Job drawing, mm, ordinate dimensions from the low corner. One solid piece. Coordinates: 2 decimals unless noted, no trailing zeros. Loops run counter-clockwise (first coordinate to the right, second up) from the corner with the lowest first, then second, coordinate; pieces in that order, holes last. Notation, with made-up numbers: M 31,-38 L 69,-38 A21 ccw 69,-27 Z; hole C 25,37 d9. An arc over 180 degrees is marked long. Answer as a JSON object with one key per item and string values. Group by question number.
1. Mould opens along X. For the marked faces 1, 2, 3 and 4 say: released by +X, released by -X, zero draft, split by the parting line, or undercut.
2. Saw through at B-B on y = 0.55. Write the cut outline in (x, z).
3. Saw through at C-C on x = 5.25. Write the cut outline in (y, z), then the cut area to 3 significant figures.
4. Drill centre lines: L1, parallel to X at y = 0.2, z = 9.25; L2, parallel to X at y = 2.65, z = 9 (1 decimal); L3, parallel to Z at x = 4.5, y = 1.4 (1 decimal). Where is each one in solid material? Low to high.
5. Saw through at A-A on x = 4.15. Write the cut outline in (y, z), then the cut area to 3 significant figures.
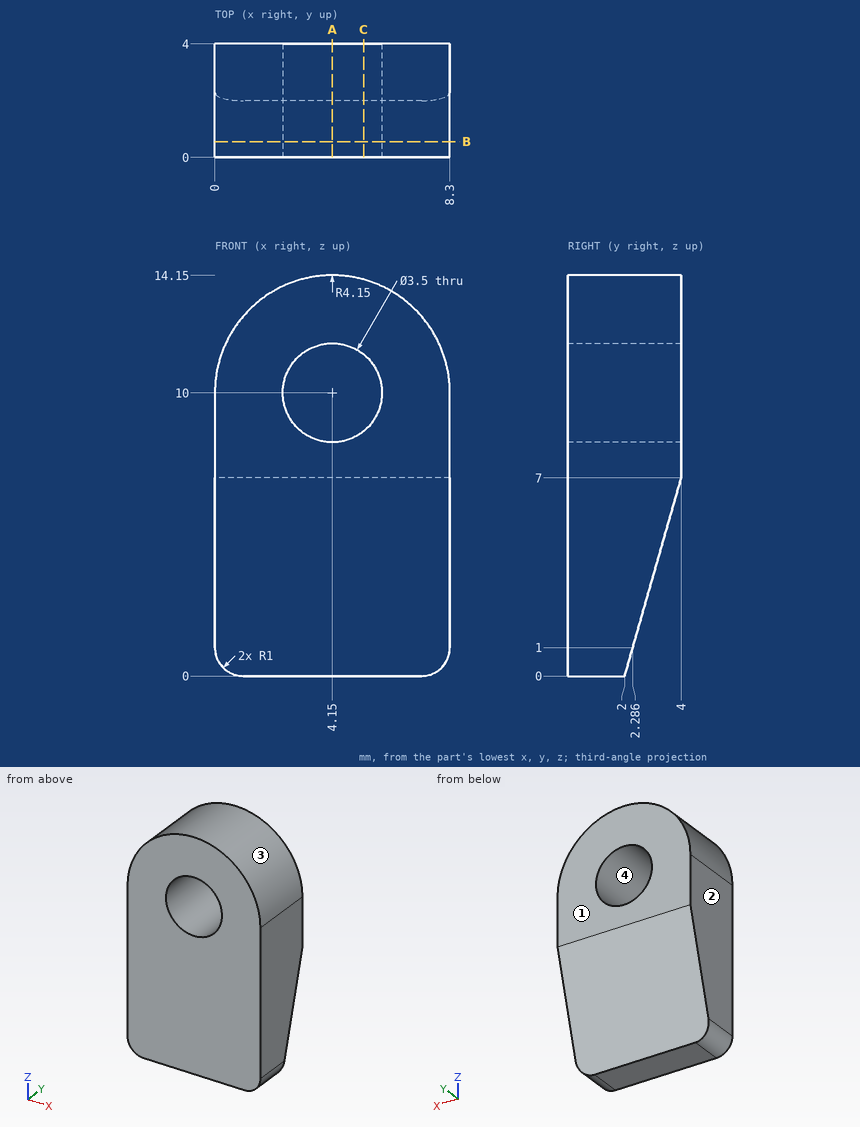
Outcome:
{
 "1": {"face 1": "zero draft", "face 2": "released by -X", "face 3": "split by the parting line", "face 4": "undercut"},
 "2": {"outline": "M 0,1 A1 ccw 1,0 L 7.3,0 A1 ccw 8.3,1 L 8.3,10 A4.15 ccw 0,10 Z; hole C 4.15,10 d3.5"},
 "3": {"outline": "M 0,0 L 2,0 L 4,7 L 4,8.64 L 0,8.64 Z; M 0,11.36 L 4,11.36 L 4,14 L 0,14 Z", "area": "38.1 mm²"},
 "4": {"L1": "x = 0 to 2.57, 5.73 to 8.3", "L2": "x = 0 to 2.7, 5.6 to 8.3", "L3": "z = 0 to 8.3, 11.7 to 14.1"},
 "5": {"outline": "M 0,0 L 2,0 L 4,7 L 4,8.25 L 0,8.25 Z; M 0,11.75 L 4,11.75 L 4,14.15 L 0,14.15 Z", "area": "35.6 mm²"}
}
